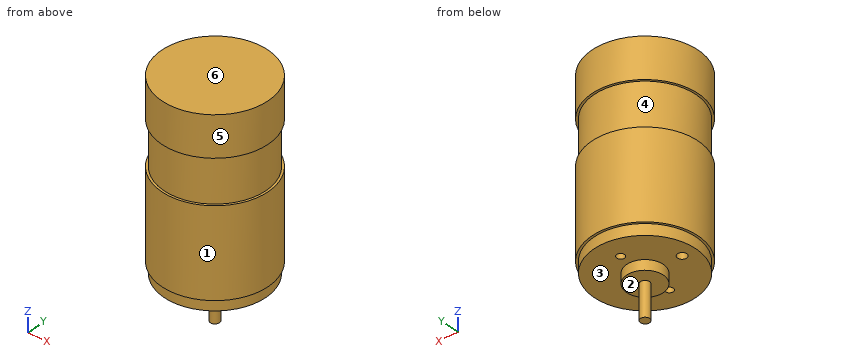
Autodesk Inventor part; units mm, degrees
ref_plane "YZ Plane" through (0, 0, 0) normal (1, 0, 0) x (0, 1, 0)
ref_plane "XZ Plane" through (0, 0, 0) normal (0, 1, 0) x (-1, 0, 0)
ref_plane "XY Plane" through (0, 0, 0) normal (0, 0, 1) x (1, 0, 0)
sketch "スケッチ1" plane through (0, 0, 0) normal (0, 0, 1) x (1, 0, 0)
  circle A0 centre (0, 0) radius 1.25
  dimension "d0" = 2.5
extrude "押し出し1" add sketch "スケッチ1" along normal blind 9.3
sketch "スケッチ2" plane through (0, 0, 9.3) normal (0, 0, 1) x (1, 0, 0)
  circle A0 centre (0, 0) radius 5
  dimension "d3" = 10
extrude "押し出し2" add sketch "スケッチ2" along normal blind 2.7
sketch "スケッチ3" plane through (0, 0, 12) normal (0, 0, 1) x (1, 0, 0)
  circle A0 centre (0, 0) radius 5
  circle A1 centre (0, 0) radius 13.9
  dimension "d6" = 27.8
extrude "押し出し3" add sketch "スケッチ3" along normal blind 3 contours A0 | A1
sketch "スケッチ4" plane through (0, 0, 15) normal (0, 0, 1) x (1, 0, 0)
  circle A0 centre (0, 0) radius 1.25
  circle A1 centre (0, 0) radius 14.5
  dimension "d9" = 29
extrude "押し出し4" add sketch "スケッチ4" along normal blind 24 contours A0 | A1
sketch "スケッチ5" plane through (0, 0, 39) normal (0, 0, 1) x (1, 0, 0)
  circle A0 centre (0, 0) radius 13.9
  dimension "d12" = 27.8
extrude "押し出し5" add sketch "スケッチ5" along normal blind 12
sketch "スケッチ6" plane through (0, 0, 51) normal (0, 0, 1) x (1, 0, 0)
  circle A0 centre (0, 0) radius 14.5
  dimension "d15" = 29
extrude "押し出し6" add sketch "スケッチ6" along normal blind 11
sketch "スケッチ7" plane through (0, 0, 12) normal (0, 0, -1) x (-1, 0, 0)
  point P0 (0, 0)
  point P1 (0, -8)
  point P2 (0, 8)
  dimension "d18" = 16
  dimension "d19" = 8
hole "穴1" at (0, -8, 12) at (0, 8, 12) direction (0, 0, 1) diameter 2.1129 depth 3 tip angle 118
sketch "スケッチ8" plane through (0, 0, 12) normal (0, 0, -1) x (-1, 0, 0)
  circle A0 centre (10, 0) radius 1.25
  point P0 (0, 0)
  dimension "d27" = 2.5
  dimension "d28" = 10
extrude "押し出し7" cut sketch "スケッチ8" against normal blind 3
properties part number "RD008_モータ(DMN29)" material "鉄、鋳鉄"
Build history of the part. All positions in model axes, mm. Face numbers are marked on the shaded views. A direction names the side the tool comes from. Round coordinates to 2 decimals unless told otherwise and drop trailing zeros. Write each loop counter-clockwise with the first axis right and the second up, starting at its lowest first coordinate (ties: lowest second). Pieces come first, ordered by that corner, then holes.
1) Band-saw the part on C-C, the plane y = 4. List the corners of the cut face in (x, z), and give its area (3 significant figures).
2) Band-saw the part on A-A, the plane x = 7.75. List the corners of the cut face in (y, z).
3) Band-saw the part on D-D, the plane x = -3.25. List the corners of the cut face in (y, z).
4) Pin check, flat tips, straight feed: pin 1 (14.5 mm diameter, centred on x = -3.5, y = -5, fed in from -Z); pin 2 (6 mm diameter, centred on x = 8, z = 35.5, fed in from -Y); pin 3 (8 mm diameter, centred on x = 8, z = 30, fed in from -Y); pin 4 (2.5 mm diameter, centred on x = 0, y = -8, fed in from -Z). Stop position of each tip, or through.
5) 3-axis set-ups, long thin cutter, end or side, ignore diameter. For the marked faces 1 and 2: which of +Z, -Z, +X, -X, +Y, -Y reach the whole face in a straight line?
6) Band-saw the part on B-B, the plane z = 48.5. List the corners of the cut face in (x, y).
7) Drill centre lines: probe 1 along Y at (x, z) = (0, 13.7); probe 2 along Z at (x, y) = (7, 12.5); probe 3 along Z at (x, y) = (0.75, 10.75). Where is each one in solid material? Low to high.
8) Mould opens along Z. For the marked faces 3, 4, 5 and 6 say: +Z half, -Z half, draft (parallel to the pull), parting line (faces both ways), or undercut.
Ans:
1. outline: (-13.94, 15) - (-13.31, 15) - (-13.31, 12) - (-3, 12) - (-3, 9.3) - (3, 9.3) - (3, 12) - (13.31, 12) - (13.31, 15) - (13.94, 15) - (13.94, 39) - (13.31, 39) - (13.31, 51) - (13.94, 51) - (13.94, 62) - (-13.94, 62) - (-13.94, 51) - (-13.31, 51) - (-13.31, 39) - (-13.94, 39) - close
1. area: 1,390 mm2
2. outline: (-12.26, 15) - (-11.54, 15) - (-11.54, 12) - (11.54, 12) - (11.54, 15) - (12.26, 15) - (12.26, 39) - (11.54, 39) - (11.54, 51) - (12.26, 51) - (12.26, 62) - (-12.26, 62) - (-12.26, 51) - (-11.54, 51) - (-11.54, 39) - (-12.26, 39) - close
3. outline: (-14.13, 15) - (-13.51, 15) - (-13.51, 12) - (-3.8, 12) - (-3.8, 9.3) - (3.8, 9.3) - (3.8, 12) - (13.51, 12) - (13.51, 15) - (14.13, 15) - (14.13, 39) - (13.51, 39) - (13.51, 51) - (14.13, 51) - (14.13, 62) - (-14.13, 62) - (-14.13, 51) - (-13.51, 51) - (-13.51, 39) - (-14.13, 39) - close
4. pin 1: stops at z = 0
4. pin 2: stops at y = -13.61
4. pin 3: stops at y = -13.94
4. pin 4: stops at z = 12
5. face 1: +Z, -Z
5. face 2: -Z
6. outline: circle Ø27.8 at (0, 0)
7. probe 1: y = -13.9 to -9.06, -6.94 to 6.94, 9.06 to 13.9
7. probe 2: z = 15 to 39, 51 to 62
7. probe 3: z = 12 to 62
8. face 3: -Z half
8. face 4: undercut
8. face 5: draft
8. face 6: +Z half
